Answer from the drawing. Dimensions are ordinates in mm from the lowest x, y and z of the part. A direction names the side the tool comes from. Coordinates: 2 decimals unless noted, no trailing zeros. Order: outer loops, then holes, each group sorted by start corner. A loop starts at its lowest first (then second) coordinate and runs counter-clockwise, first axis right, second up. Notation, with made-up numbers: (52, 54.25) -> (73, 54.25) arc R34 cw to (73, 87.25) -> close; hole circle Ø6 at (43, 55.25). An arc over 180 degrees is marked (long way). Answer in a Markdown table with one row per item.
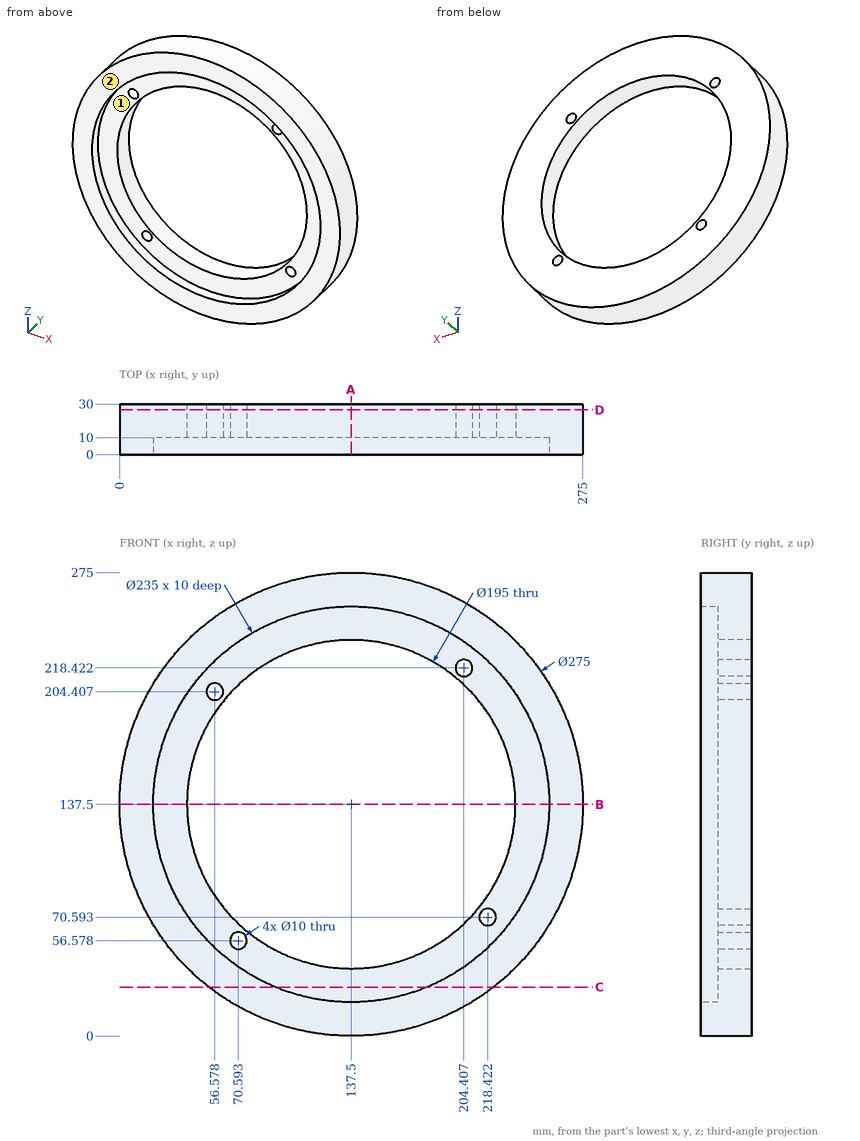
Q1. The part is cut by section C-C (z = 29). Write down the section's boundary in (x, y).
Outcome:
| item | result |
|---|---|
| outline | (53.04, 0) -> (92.4, 0) -> (92.4, 10) -> (182.6, 10) -> (182.6, 0) -> (221.96, 0) -> (221.96, 30) -> (53.04, 30) -> close |
Q2. The part is cut by section A-A (x = 137.5). Write down the section's boundary in (y, z), then the cut area to 3 significant figures.
Outcome:
| item | result |
|---|---|
| outline | (0, 0) -> (30, 0) -> (30, 40) -> (10, 40) -> (10, 20) -> (0, 20) -> close; (0, 255) -> (10, 255) -> (10, 235) -> (30, 235) -> (30, 275) -> (0, 275) -> close |
| area | 2,000 mm² |
Q3. The part is cut by section B-B (z = 137.5). Write down the section's boundary in (x, y).
Outcome:
| item | result |
|---|---|
| outline | (0, 0) -> (20, 0) -> (20, 10) -> (40, 10) -> (40, 30) -> (0, 30) -> close; (235, 10) -> (255, 10) -> (255, 0) -> (275, 0) -> (275, 30) -> (235, 30) -> close |
Q4. Consider line 1 (Z direction, x = 204.5, y = 23.5) (1 decimal); line 2 (X direction, y = 20, z = 137.5); line 3 (X direction, y = 5.75, z = 185) (1 decimal). Determine where each line is inside the solid, lowest interval first.
Outcome:
| item | result |
|---|---|
| line 1 | 17.4 to 66.7, 208.3 to 213.4, 223.4 to 257.6 |
| line 2 | 0 to 40, 235 to 275 |
| line 3 | 8.5 to 30, 245 to 266.5 |
Q5. For the marked faces 1 and 2, determine the directions among +Z, -Z, +X, -X, +Y, -Y from which every point of the face is accessible in a straight line to the end or side of a thin tool.
Outcome:
| item | result |
|---|---|
| face 1 | -Y |
| face 2 | +Z, -Z, +X, -X, -Y |
Q6. The part is cut by section D-D (y = 26.5). Write down the section's boundary in (x, z).
Outcome:
| item | result |
|---|---|
| outline | circle Ø275 at (137.5, 137.5); hole circle Ø195 at (137.5, 137.5); hole circle Ø10 at (56.58, 204.41); hole circle Ø10 at (70.59, 56.58); hole circle Ø10 at (204.41, 218.42); hole circle Ø10 at (218.42, 70.59) |
Q7. Given pin 1 (6 mm diameter, centred on x = 79.5, y = 9, fed in from -Z); pin 2 (13 mm diameter, centred on x = 56.58, z = 204.41, fed in from +Y); pin 3 (10 mm diameter, centred on x = 46, y = 3.5, fed in from -Z); pin 4 (8 mm diameter, centred on x = 196, y = 16, fed in from -Z), each flat-ended and moving along its own axis, determine where each tip first touches the part or whether it passes through.
Outcome:
| item | result |
|---|---|
| pin 1 | z = 11.48 |
| pin 2 | y = 30 |
| pin 3 | z = 30.62 |
| pin 4 | z = 11.26 |
